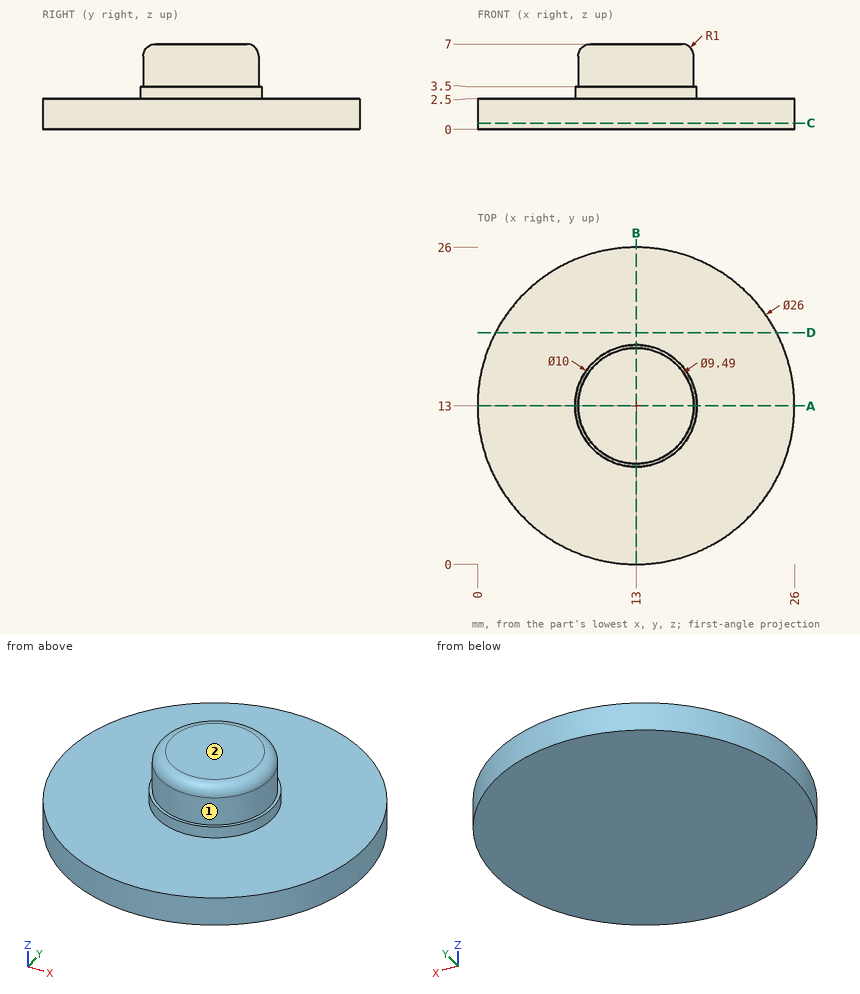
Check sheet for the drawn part. Datum: minimum x, y, z corner. Units: mm. A direction names the side the tool comes from. Coordinates: 2 decimals unless noted, no trailing zeros. Loops run counter-clockwise (first coordinate to the right, second up) from the corner with the lowest first, then second, coordinate; pieces in that order, holes last. Notation, with made-up numbers: M -4.5,68.25 L 33.5,68.25 A23 ccw 33.5,80.25 Z; hole C 40,-27 d11. An arc over 180 degrees is marked long. Answer as a JSON object with one key per item and string values.
1. Sectioned sample at C-C on z = 0.5. Record the cut outline in (x, y).
Outcome:
{"outline": "C 13,13 d26"}
2. Scan lines: L1, parallel to Z at x = 20.75, y = 11.5; L2, parallel to X at y = 1, z = 0.5; L3, parallel to X at y = 2.75, z = 1.5. Record each from-to range of solid material in increasing order. Write a range as from..to.
Outcome:
{"L1": "0..2.5", "L2": "8..18", "L3": "5..21"}
3. Sectioned sample at A-A on y = 13. Record the cut outline in (x, z) (3 decimals), and give its area (3 significant figures).
Outcome:
{"outline": "M 0,0 L 26,0 L 26,2.5 L 18,2.5 L 18,3.5 L 17.745,3.5 L 17.745,6 A1 ccw 16.745,7 L 9.255,7 A1 ccw 8.255,6 L 8.255,3.5 L 8,3.5 L 8,2.5 L 0,2.5 Z", "area": "108 mm²"}
4. Depth check by flat-ended pin: P1, Ø4, axis at y = 14, z = 3, coming from the +X side; P2, Ø1.5, axis at y = 16.5, z = 2, coming from the +X side; P3, Ø1.5, axis at x = 9, z = 2.5, coming from the -Y side. Enter the tip coordinate at first touch or a pass-through.
Outcome:
{"P1": "x = 26", "P2": "x = 25.71", "P3": "y = 0.41"}
5. Access from +Z, -Z, +X, -X, +Y, -Y to the whole of each face (thin tool, end or side, straight path). Record for the marked faces 1 and 2.
Outcome:
{"face 1": "+Z", "face 2": "+Z, +X, -X, +Y, -Y"}
6. Sectioned sample at D-D on y = 19. Record the cut outline in (x, z).
Outcome:
{"outline": "M 1.47,0 L 24.53,0 L 24.53,2.5 L 1.47,2.5 Z"}
